Work out the finished part from the listing and answer in its coordinate system (mm). A direction names the side the tool comes from. Give positions to 0.01 mm unless a question says otherwise; leave off trailing zeros. Loops run counter-clockwise (first coordinate to the right, second up) from the corner with the lowest first, then second, coordinate; pieces in that order, holes last. Notation, with made-up numbers: (4, 78.5) - (20, 78.5) arc R19 ccw to (20, 113.5) - close; hole circle Ø6 at (67.25, 78). An arc over 180 degrees is marked (long way). One line per item, written item: value.
from build123d import *

# Parameters (mm, degrees)
SKETCH1_R           = 0.9
BOSS_EXTRUDE1_DEPTH = 4
SKETCH2_W           = 16.2
SKETCH2_H           = 21.74
CUT_EXTRUDE1_DEPTH  = 2


with BuildPart() as part:
    # Sketch1 → Boss-Extrude1 (new body)
    with BuildSketch(Plane.XY):
        with BuildLine():
            Line((0, 14.74), (0, 7))
            Line((0, 7), (4, 7))
            Line((4, 7), (4, 5))
            Line((4, 5), (0, 5))
            Line((0, 5), (0, 2))
            ThreePointArc((0, 2), (0.585786438, 0.585786438), (2, 0))
            Line((2, 0), (14.2, 0))
            ThreePointArc((14.2, 0), (15.614213562, 0.585786438), (16.2, 2))
            Line((16.2, 2), (16.2, 5))
            Line((16.2, 5), (12.2, 5))
            Line((12.2, 5), (12.2, 7))
            Line((12.2, 7), (16.2, 7))
            Line((16.2, 7), (16.2, 14.74))
            Line((16.2, 14.74), (12.2, 14.74))
            Line((12.2, 14.74), (12.2, 16.74))
            Line((12.2, 16.74), (16.2, 16.74))
            Line((16.2, 16.74), (16.2, 19.74))
            ThreePointArc((16.2, 19.74), (15.614213562, 21.154213562), (14.2, 21.74))
            Line((14.2, 21.74), (2, 21.74))
            ThreePointArc((2, 21.74), (0.585786438, 21.154213562), (0, 19.74))
            Line((0, 19.74), (0, 16.74))
            Line((0, 16.74), (4, 16.74))
            Line((4, 16.74), (4, 14.74))
            Line((4, 14.74), (0, 14.74))
        make_face()
        with Locations((13.45, 2.5)):
            Circle(SKETCH1_R, mode=Mode.SUBTRACT)
        with Locations((2.75, 19.24)):
            Circle(SKETCH1_R, mode=Mode.SUBTRACT)
        with Locations((2.75, 2.5)):
            Circle(SKETCH1_R, mode=Mode.SUBTRACT)
        with Locations((13.45, 19.24)):
            Circle(SKETCH1_R, mode=Mode.SUBTRACT)
    extrude(amount=BOSS_EXTRUDE1_DEPTH)

    # Sketch2 → Cut-Extrude1 (cut)
    with BuildSketch(Plane(origin=(0, 0, 0), x_dir=(-1, 0, 0), z_dir=(0, 0, -1))):
        with Locations((-8.1, 10.87)):
            Rectangle(SKETCH2_W, SKETCH2_H)
    extrude(amount=-CUT_EXTRUDE1_DEPTH, mode=Mode.SUBTRACT)


solid = part.part
1. The mould has two halves that part along X. Classify faces 1 (the flat face through (8, 11, 4)), 2 (the cylindrical face through (2.555, 18.361, 2.986)), 3 (the cylindrical face through (0.57, 0.6, 2.99)): released by +X, released by -X, zero draft, split by the parting line, or undercut.
Output:
face 1: zero draft
face 2: undercut
face 3: released by -X
2. Section A-A (y = 2.5) is taken. Write down the section's boundary in (x, z).
Output:
outline: (0, 2) - (1.85, 2) - (1.85, 4) - (0, 4) - close; (3.65, 2) - (12.55, 2) - (12.55, 4) - (3.65, 4) - close; (14.35, 2) - (16.2, 2) - (16.2, 4) - (14.35, 4) - close
3. Section C-C (x = 13.45) is taken. Write down the section's boundary in (y, z).
Output:
outline: (0, 2) - (1.6, 2) - (1.6, 4) - (0, 4) - close; (3.4, 2) - (5, 2) - (5, 4) - (3.4, 4) - close; (7, 2) - (14.74, 2) - (14.74, 4) - (7, 4) - close; (16.74, 2) - (18.34, 2) - (18.34, 4) - (16.74, 4) - close; (20.14, 2) - (21.74, 2) - (21.74, 4) - (20.14, 4) - close
4. Section B-B (z = 2.5) is taken. Write down the section's boundary in (x, y).
Output:
outline: (0, 2) arc R2 ccw to (2, 0) - (14.2, 0) arc R2 ccw to (16.2, 2) - (16.2, 5) - (12.2, 5) - (12.2, 7) - (16.2, 7) - (16.2, 14.74) - (12.2, 14.74) - (12.2, 16.74) - (16.2, 16.74) - (16.2, 19.74) arc R2 ccw to (14.2, 21.74) - (2, 21.74) arc R2 ccw to (0, 19.74) - (0, 16.74) - (4, 16.74) - (4, 14.74) - (0, 14.74) - (0, 7) - (4, 7) - (4, 5) - (0, 5) - close; hole circle Ø1.8 at (2.75, 2.5); hole circle Ø1.8 at (2.75, 19.24); hole circle Ø1.8 at (13.45, 2.5); hole circle Ø1.8 at (13.45, 19.24)
5. For faces 4 (the flat face through (14, 16.74, 3)), 5 (the flat face through (2, 5, 3)), 6 (the cylindrical face through (13.255, 18.361, 2.986)), determine the directions among +Z, -Z, +X, -X, +Y, -Y from which every point of the face is accessible in a straight line to the end or side of a thin tool.
Output:
face 4: +Z, -Z, +X
face 5: +Z, -Z, -X
face 6: +Z, -Z
6. Find the intervals of material crossed by line 1 along X through (y, z) = (19.24, 2.6); line 2 along Y through (x, z) = (13.45, 2.95); line 3 along Y through (x, z) = (2, 3.2), in increasing order.
Output:
line 1: x = 0 to 1.85, 3.65 to 12.55, 14.35 to 16.2
line 2: y = 0 to 1.6, 3.4 to 5, 7 to 14.74, 16.74 to 18.34, 20.14 to 21.74
line 3: y = 0 to 2, 3 to 5, 7 to 14.74, 16.74 to 18.74, 19.74 to 21.74
7. Section D-D (x = 1) is taken. Write down the section's boundary in (y, z).
Output:
outline: (0.27, 2) - (5, 2) - (5, 4) - (0.27, 4) - close; (7, 2) - (14.74, 2) - (14.74, 4) - (7, 4) - close; (16.74, 2) - (21.47, 2) - (21.47, 4) - (16.74, 4) - close
8. Flat-ended cylindrical pins translate along their axes: pin 1 Ø1 at (x, z) = (1, 3) entering from +Y; pin 2 Ø0.6 at (y, z) = (16, 3) entering from -X; pin 3 Ø1 at (y, z) = (15.5, 3) entering from +X; pin 4 Ø1.6 at (x, y) = (2.75, 2.5) entering from +Z. Find the tip coordinate at first contact, or state that the pin passes through.
Output:
pin 1: stops at y = 21.68
pin 2: stops at x = 4
pin 3: stops at x = 12.2
pin 4: passes through
